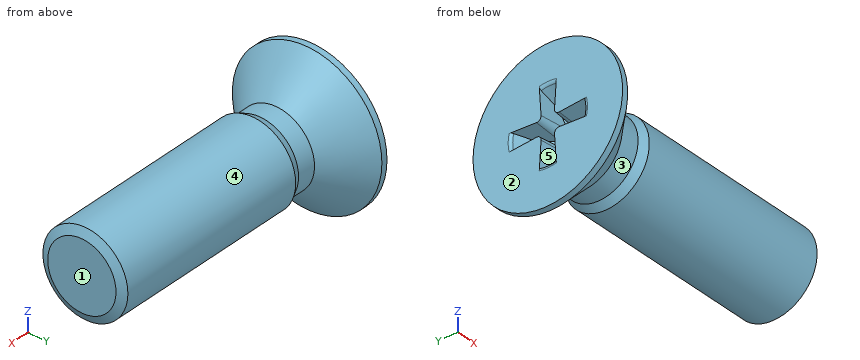
Autodesk Inventor part; units mm, degrees
ref_plane "Work Plane2" through (3.35, 0, 0) normal (0, 0, -1) x (1, 0, 0)
ref_plane "YZ Plane" through (0, 0, 0) normal (1, 0, 0) x (0, 1, 0)
ref_plane "XZ Plane" through (0, 0, 0) normal (0, 1, 0) x (-1, 0, 0)
sketch "Sketch1" plane through (0, 0, 0) normal (0, 0, 1) x (1, 0, 0)
  line L0 (2.05, 0) -> (16, 0)
  line L1 (16, 0) -> (16, 2.5)
  line L2 (16, 2.5) -> (4.1, 2.5)
  line L3 (4.1, 2.5) -> (3.6092, 2.2546)
  line L4 (3.6092, 2.2546) -> (2.5, 2.2546)
  line L5 (0, 4.4) -> (0, 2.21)
  line L6 (0, 2.21) -> (1.1905, 1.6164)
  line L7 (1.1905, 1.6164) -> (2.05, 0)
  line L8 (-3.2, 0) -> (19.2, 0)
  line L9 (0, -0.88) -> (0, 5.28)
  line L10 (0, 4.4) -> (0.3546, 4.4)
  line L11 (0.3546, 4.4) -> (2.5, 2.2546)
  line L12 (4.1, 2.5) -> (2.2546, 2.5) construction
  dimension "d1" = 11.9
  dimension "d2" = 5
  dimension "d3" = 4.5092
  dimension "d4" = 4.42
  dimension "d5" = 26.5
  dimension "d6" = 62
  dimension "d7" = 2.05
  dimension "d8" = 0.4908
  dimension "d12" = 8.8
  dimension "d13" = 45
  dimension "d15" = 16
  dimension "d24" = 2.5
revolve "Body" add sketch "Sketch1" angle 360 about axis through (2.05, 0, 0) along (1, 0, 0) contours L7 L6 L5 L10 L11 L4 L3 L2 L1 L0
sketch "Sketch2" plane through (0, 0, 0) normal (-1, 0, 0) x (0, 0, 1)
  line L0 (0, 2.21) -> (0, 0) construction
  line L1 (0, 0) -> (2.21, 0) construction
  arc A0 (0.663, 0) -> (0, 0.663) centre (0, 0) ccw construction
  arc A1 (0.7735, 0) -> (0, 0.7735) centre (0, 0) ccw construction
  arc A2 (2.1539, 0.495) -> (0.495, 2.1539) centre (0, 0) ccw
  line L2 (0, 0) -> (1.5627, 1.5627) construction
  line L3 (0.495, 2.1539) -> (0.3952, 0.6649)
  line L4 (2.1539, 0.495) -> (0.6649, 0.3952)
  arc A3 (0.495, 2.1539) -> (0, 2.21) centre (0, 0) ccw
  arc A4 (2.21, 0) -> (2.1539, 0.495) centre (0, 0) ccw
  line L5 (0, -6.16) -> (0, 6.16)
  line L6 (-6.16, 0) -> (6.16, 0)
  arc A5 (0.495, -2.1539) -> (2.1539, -0.495) centre (0, 0) ccw
  line L7 (0.495, -2.1539) -> (0.3952, -0.6649)
  line L8 (2.1539, -0.495) -> (0.6649, -0.3952)
  arc A6 (0, -2.21) -> (0.495, -2.1539) centre (0, 0) ccw
  arc A7 (2.1539, -0.495) -> (2.21, 0) centre (0, 0) ccw
  arc A8 (-0.495, 2.1539) -> (-2.1539, 0.495) centre (0, 0) ccw
  line L9 (-0.495, 2.1539) -> (-0.3952, 0.6649)
  line L10 (-2.1539, 0.495) -> (-0.6649, 0.3952)
  arc A9 (0, 2.21) -> (-0.495, 2.1539) centre (0, 0) ccw
  arc A10 (-2.1539, 0.495) -> (-2.21, 0) centre (0, 0) ccw
  arc A11 (-0.495, -2.1539) -> (0, -2.21) centre (0, 0) ccw
  arc A12 (-2.1539, -0.495) -> (-0.495, -2.1539) centre (0, 0) ccw
  arc A13 (-2.21, 0) -> (-2.1539, -0.495) centre (0, 0) ccw
  line L11 (-2.1539, -0.495) -> (-0.6649, -0.3952)
  line L12 (-0.495, -2.1539) -> (-0.3952, -0.6649)
  arc A14 (0.3952, 0.6649) -> (0.6649, 0.3952) centre (0.648, 0.648) ccw
  arc A15 (0.6649, -0.3952) -> (0.3952, -0.6649) centre (0.648, -0.648) ccw
  arc A16 (-0.6649, 0.3952) -> (-0.3952, 0.6649) centre (-0.648, 0.648) ccw
  arc A17 (-0.3952, -0.6649) -> (-0.6649, -0.3952) centre (-0.648, -0.648) ccw
  point P0 (1.5627, -1.5627)
  point P1 (-1.5627, 1.5627)
  point P2 (-1.5627, -1.5627)
  dimension "d17" = 1.326
  dimension "d18" = 1.547
  dimension "d19" = 4.42
  dimension "d20" = 45
  dimension "d21" = 0.495
extrude "Slot" add sketch "Sketch2" against normal up to next draft 5 contours L4 A14 L3 A2 | A5 L7 A15 L8 | L9 A16 L10 A8 | A12 L11 A17 L12
fillet "Fillet1" radius 0.198 4 edges at (0, 2.21, 0) (0, 0, -2.21) (0, -2.21, 0) (0, 0, 2.21)
thread "Thread"
chamfer "Chamfer1" distance 0.4908 distance2 0.2454 1 edges at (16, -2.5, 0) measured on face at (16, 0.2278, 0.5045)
ref_plane "Work Plane2" through (3.35, 0, 0) normal (0, 0, -1) x (1, 0, 0)
equation "\"d1\" = GEL"
equation "\"d2\" = GD"
equation "\"d3\" = BDM"
equation "\"d4\" = SDM"
equation "\"d7\" = INTI"
equation "\"d8\" = GAL"
equation "\"d12\" = KOD"
equation "\"d13\" = 0.5 * SEWI"
equation "\"d15\" = NLG"
equation "\"d24\" = KOH"
equation "\"d17\" = 0.3 * SDM"
equation "\"d18\" = 0.35 * SDM"
equation "\"d19\" = SDM"
equation "\"d21\" = 0.5 * SBR"
equation "\"d23\" = 0.2 * SBR"
equation "\"d10\" = GEL"
equation "\"d25\" = -0.5 * SPD + 0.5 * GD"
equation "\"d26\" = 0.5 * GAL"
equation "\"NLG\" = 16"
equation "\"GEL\" = 11.9"
equation "\"GAL\" = 0.61345 * PTC"
equation "\"SPD\" = NND - 1.2269 * PTC"
equation "\"KOD\" = 8.8"
equation "\"KOH\" = 2.5"
equation "\"SBR\" = 0.99"
equation "\"INTI\" = 2.05"
equation "\"SDM\" = 4.42"
equation "\"GD\" = NND"
equation "\"BDM\" = NND - GAL"
equation "\"SEWI\" = 90deg"
equation "\"d9\" = SDM"
equation "\"GUL\" = 0.61345 * PTC"
equation "\"TOA\" = 30deg"
equation "\"EPV\" = 5"
equation "\"THREADDIA\" = 5"
equation "\"RR\" = 0.5"
equation "\"PTC\" = 0.8"
equation "\"NND\" = 5"
equation "\"GD1\" = THREADDIA - 1.2269 * PTC"
properties part number "AS 1427 - M5 x 16" material "Steel, Mild"
Geometry: final body of the model. Coordinates: model frame, mm. Face numbers are marked on the shaded views. A direction names the side the tool comes from. Coordinates: 2 decimals unless noted, no trailing zeros. Write each loop counter-clockwise with the first axis right and the second up, starting at its lowest first coordinate (ties: lowest second). Pieces come first, ordered by that corner, then holes. Notation, with made-up numbers: M 56,-8.5 L 91,-8.5 A3 cw 91,-4.5 Z; hole C -22.5,24 d8. An arc over 180 degrees is marked long. Answer as CSV lines item,"result". Start each with the question number.
Q1. Pin query (flat end, axial travel): P1, Ø3, axis at x = 8.5, z = 3.5, coming from the -Y side; P2, Ø4, axis at x = 9.5, y = 1, coming from the +Z side. Return the tip coordinate at first contact, or that it passes through.
Q2. Mould query, pull axis X, two halves, no side actions, for the marked faces 1, 2 and 3. Classes: released by +X, released by -X, zero draft, split by the parting line, or undercut.
Q3. Line query: line 1 (Z direction, x = 7.75, y = 0); line 2 (X direction, y = 3, z = -2.75); line 3 (Z direction, x = 3.75, y = -0.75). Output: solid intervals per line, ascending. Write a range as from..to.
Q4. Reachability of the marked faces 4 and 5 from +Z, -Z, +X, -X, +Y, -Y: full face, straight path, thin tool, end or side. Return the list, or none.
Q5. Cut plane A-A on x = 12.75. Return the cut outline in (y, z), then the cut area to 3 significant figures.
Q6. Cut plane B-B on x = 2.75. Return the cut outline in (y, z), then the cut area to 3 significant figures.
Findings below:
1,P1,"stops at y = -1.5"
1,P2,"stops at z = 2.5"
2,face 1,"released by +X"
2,face 2,"released by -X"
2,face 3,"undercut"
3,line 1,"z = -2.5..2.5"
3,line 2,"x = 0..0.68"
3,line 3,"z = -2.2..2.2"
4,face 4,"+X"
4,face 5,"-X"
5,outline,"C 0,0 d5"
5,area,"19.6 mm2"
6,outline,"C 0,0 d4.51"
6,area,"16.0 mm2"
